Geometry check sheet. Reference: the model listing, model coordinates, mm. A direction names the side the tool comes from. Give positions to 0.01 mm unless a question says otherwise; leave off trailing zeros. Write each loop counter-clockwise with the first axis right and the second up, starting at its lowest first coordinate (ties: lowest second). Pieces come first, ordered by that corner, then holes. Notation, with made-up numbers: M 89,72.5 L 147,72.5 A15 cw 147,97.5 Z; hole C 17.5,52.5 d2. An arc over 180 degrees is marked long. Write each question's results on one line, items separated by ' | '.
Autodesk Inventor part; units mm, degrees
ref_plane "YZ Plane" through (0, 0, 0) normal (1, 0, 0) x (0, 1, 0)
ref_plane "XZ Plane" through (0, 0, 0) normal (0, 1, 0) x (-1, 0, 0)
ref_plane "XY Plane" through (0, 0, 0) normal (0, 0, 1) x (1, 0, 0)
sketch "Boceto1" plane through (0, 0, 0) normal (0, 0, 1) x (1, 0, 0)
  circle A0 centre (0, 0) radius 18
  circle A1 centre (0, 0) radius 20
  line L0 (0, -20) -> (40, -20)
  line L1 (40, -20) -> (40, -30)
  line L2 (40, -30) -> (0, -30)
  line L3 (0, -30) -> (-40, -30)
  line L4 (-40, -30) -> (-40, -20)
  line L5 (-40, -20) -> (0, -20)
  line L6 (-40, -30) -> (40, -30)
  line L7 (40, -30) -> (40, -110)
  line L8 (40, -110) -> (-40, -110)
  line L9 (-40, -110) -> (-40, -30)
  line L10 (0, 18) -> (0, -21.2387) construction
  circle A2 centre (0, 0) radius 20
  line L11 (20, 0) -> (20, -20)
  line L12 (-20, 0) -> (-20, -20)
  dimension "d0" = 36
  dimension "d1" = 40
  dimension "d2" = 40
  dimension "d3" = 10
  dimension "d4" = 40
  dimension "d5" = 80
extrude "Extrusión1" add sketch "Boceto1" along normal blind 10 contours A0 | A1 | L11 L0 A1 | A1 L5 L12 | L0 L1 L2 L3 L4 L5 | L7 L8 L9 L3 L2
sketch "Boceto2" plane through (0, 0, 0) normal (0, 0, -1) x (-1, 0, 0)
  circle A0 centre (0, 0) radius 18
  dimension "d9" = 36
hole "Agujero1" at (0, 0, 0) direction (0, 0, 1) diameter 36 depth 10 tip angle 118
properties part number "Soporte ensamble"
Q1. Release check for a two-part mould opening along X. For faces 4 (the face through (-1, -59, 0)), 5 (the face through (-17.847, -2.343, 5.07)), 6 (the face through (0, 20, 5)) record: released by +X, released by -X, zero draft, split by the parting line, or undercut.
Answer key:
face 4: zero draft | face 5: undercut | face 6: split by the parting line
Q2. Access from +Z, -Z, +X, -X, +Y, -Y to the whole of each face (thin tool, end or side, straight path). Record for faces 1 (the face through (40, -64, 5)), 2 (the face through (-20, -10, 5)), 3 (the face through (30, -20, 5)).
Answer key:
face 1: +Z, -Z, +X, +Y, -Y | face 2: +Z, -Z, -X, +Y | face 3: +Z, -Z, +X, +Y
Q3. Section check B-B (z = 6.5). Enter the section's corners in (x, y).
Answer key:
outline: M -40,-110 L 40,-110 L 40,-20 L 20,-20 L 20,0 A20 ccw -20,0 L -20,-20 L -40,-20 Z; hole C 0,0 d36
Q4. Section check A-A (x = 0). Enter the section's corners in (y, z).
Answer key:
outline: M -110,0 L -18,0 L -18,10 L -110,10 Z; M 18,0 L 20,0 L 20,10 L 18,10 Z
Q5. Section check C-C (y = -6.5). Enter the section's corners in (x, z).
Answer key:
outline: M -20,0 L -16.79,0 L -16.79,10 L -20,10 Z; M 16.79,0 L 20,0 L 20,10 L 16.79,10 Z
Q6. Material ranges on probe 1 along Y at (x, z) = (0, 7.75); probe 2 along X at (y, z) = (0, 5); probe 3 along Y at (x, z) = (-27.5, 6.75), recorded low to high. Write a range as [from, to].
Answer key:
probe 1: y = [-110, -18], [18, 20] | probe 2: x = [-20, -18], [18, 20] | probe 3: y = [-110, -20]
Q7. Depth check by flat-ended pin: P1, Ø3, axis at x = 30.5, z = 6, coming from the +Y side; P2, Ø3, axis at y = -5.5, z = 6.5, coming from the -X side; P3, Ø1, axis at x = 17.5, z = 1.5, coming from the +Y side. Enter the tip coordinate at first touch or a pass-through.
Answer key:
P1: stops at y = -20 | P2: stops at x = -20 | P3: stops at y = 10.54
Q8. Section check D-D (x = 22.5). Enter the section's corners in (y, z).
Answer key:
outline: M -110,0 L -20,0 L -20,10 L -110,10 Z
